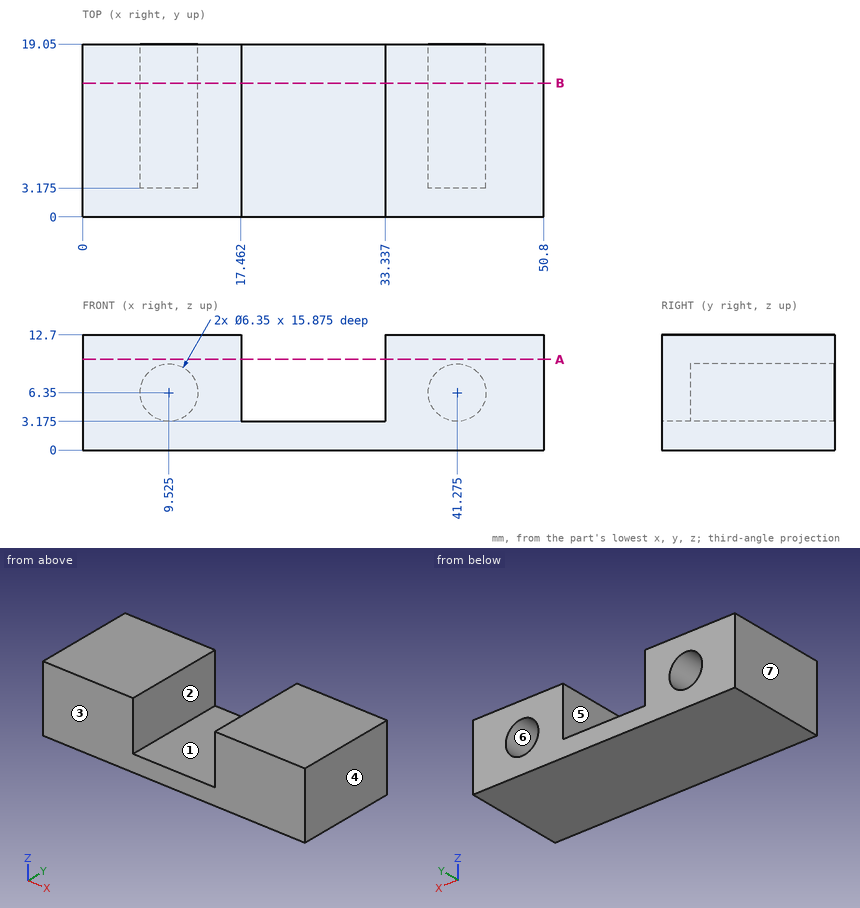
Can you work these out from the drawing? Everything is in mm from the part's minimum corner. A direction names the side the tool comes from. Coordinates: 2 decimals unless noted, no trailing zeros. Loops run counter-clockwise (first coordinate to the right, second up) from the corner with the lowest first, then second, coordinate; pieces in that order, holes last. Notation, with made-up numbers: (59, -33) - (73, -33) arc R11 cw to (73, -16) - close; hole circle Ø1 at (39, 1). An arc over 180 degrees is marked (long way). Put each result on its own line as item: value. Start each with the question number.
Item 1: If we mould it in two halves opening along X, with no side actions, what happens to the marked faces 1, 2, 3 and 4? For each: +X half, -X half, draft (parallel to the pull), parting line (faces both ways), or undercut.
Item 2: For pin 1 (8 mm diameter, centred on x = 29, y = 13.5, fed in from +Z) (1 decimal); pin 2 (5.5 mm diameter, centred on x = 9.525, z = 6.35, fed in from +Y) (1 decimal), each with a flat end and sliding along its axis, tell me the tip position at first contact or that it passes through.
Item 3: If I drill on line 1 along X through (y, z) = (7, 6.35); line 2 along X through (y, z) = (10.5, 4) (1 decimal); line 3 along X through (y, z) = (6, 10.5), over which ranges is the centre line in solid material (lowest first)?
Item 4: Suppose I cut it at B-B (y = 14.75). State how many separate pieces and enclosed holes the cut face has.
Item 5: Suppose I cut it at A-A (z = 10). Please give me the cut outline in (x, y), and give its area (3 significant figures).
Item 6: Which directions (+Z, -Z, +X, -X, +Y, -Y) give clear straight access to the entire face, cutting with the end or side of a thin tool? Please do the marked faces 5, 6 and 7.
Here are the results:
1. face 1: undercut
1. face 2: undercut
1. face 3: draft
1. face 4: +X half
2. pin 1: z = 3.2
2. pin 2: y = 3.2
3. line 1: 0 to 6.35, 12.7 to 17.46, 33.34 to 38.1, 44.45 to 50.8
3. line 2: 0 to 7.4, 11.7 to 17.5, 33.3 to 39.1, 43.4 to 50.8
3. line 3: 0 to 17.46, 33.34 to 50.8
4. separate pieces: 1
4. enclosed holes: 2
5. outline: (0, 0) - (17.46, 0) - (17.46, 19.05) - (0, 19.05) - close; (33.34, 0) - (50.8, 0) - (50.8, 19.05) - (33.34, 19.05) - close
5. area: 665 mm²
6. face 5: +Z, +Y, -Y
6. face 6: +Y
6. face 7: +Z, -Z, -X, +Y, -Y
